Check sheet for the modelled part. Datum: model origin and axes. Units: mm. A direction names the side the tool comes from. Coordinates: 2 decimals unless noted, no trailing zeros. Loops run counter-clockwise (first coordinate to the right, second up) from the corner with the lowest first, then second, coordinate; pieces in that order, holes last. Notation, with made-up numbers: M -36.5,10 L -9.5,10 A21 ccw -9.5,14 Z; hole C 61.25,51 d5. An arc over 180 degrees is marked long. Use CSV: the item, a comma, the result in double quotes. Start each with the question number.
(1) Set-up check for faces 1 (the cylindrical face through (-61.922, -104.907, 3.944)), 2 (the flat face through (-2, 120, 4)): record each of +Z, -Z, +X, -X, +Y, -Y from which the full face is reachable in a straight line by a thin tool's end or side.
(2) Scan lines: line 1 (Y direction, x = 98.5, z = 7.75); line 2 (X direction, y = 79, z = 3); line 3 (X direction, y = 106, z = 5). Record each from-to range of solid material in increasing order.
(3) Section check B-B on y = -105. Record the cut outline in (x, z).
(4) Go/stop test with a flat-tipped pin: pin 1 Ø5.5 at (x, y) = (45.58, -77.36) entering from -Z. Record where the tip stops, or that it passes through.
(5) Section check D-D on x = -16. Record the cut outline in (y, z).
(6) Section check A-A on x = 97.5. Record the cut outline in (y, z), and give its area (3 significant figures).
(7) Section check C-C on y = 0. Record the cut outline in (x, z).
(8) Draft check along X on faces 3 (the cylindrical face through (-109.943, 104.907, 3.944)), 4 (the flat face through (-55, 55, 8)), 5 (the flat face through (119.579, -2, 4)). Enter one of: pulls with the +X half, pulls with the -X half, needs draft (parallel to the pull), parting line crosses it, or undercut.
from build123d import *

# Parameters (mm, degrees)
F0_W     = 240
F0_H     = 240
F0_R     = 4.5
F0_R_2   = 65
F1_DEPTH = 8


with BuildPart() as f1:
    # F0 (on Top) → F1 (new body)
    with BuildSketch(Plane.XY):
        with Locations((-0.42114, 0)):
            Rectangle(F0_W, F0_H)
        with BuildLine():
            ThreePointArc((-105.444208, -109.5), (-109.944211, -104.994235), (-105.432677, -100.500015))
            Line((-105.432677, -100.500015), (-66.432677, -100.500015))
            ThreePointArc((-66.432677, -100.500015), (-61.921144, -105.005765), (-66.444208, -109.499941))
            Line((-66.444208, -109.499941), (-105.444208, -109.5))
        make_face(mode=Mode.SUBTRACT)
        with Locations((-46.42114, -77.356318)):
            Circle(F0_R, mode=Mode.SUBTRACT)
        with Locations((45.57886, -77.356318)):
            Circle(F0_R, mode=Mode.SUBTRACT)
        with BuildLine():
            ThreePointArc((64.555792, -109.5), (60.055789, -104.994235), (64.567323, -100.500015))
            Line((64.567323, -100.500015), (103.567323, -100.500015))
            ThreePointArc((103.567323, -100.500015), (108.078856, -105.005765), (103.555792, -109.499941))
            Line((103.555792, -109.499941), (64.555792, -109.5))
        make_face(mode=Mode.SUBTRACT)
        with BuildLine():
            ThreePointArc((-105.444208, 100.5), (-109.944211, 105.005765), (-105.432677, 109.499985))
            Line((-105.432677, 109.499985), (-66.432677, 109.499985))
            ThreePointArc((-66.432677, 109.499985), (-61.921144, 104.994235), (-66.444208, 100.500059))
            Line((-66.444208, 100.500059), (-105.444208, 100.5))
        make_face(mode=Mode.SUBTRACT)
        with Locations((-46.42114, 77.356318)):
            Circle(F0_R, mode=Mode.SUBTRACT)
        with Locations((-0.42114, 0)):
            Circle(F0_R_2, mode=Mode.SUBTRACT)
        with Locations((45.57886, 77.356318)):
            Circle(F0_R, mode=Mode.SUBTRACT)
        with BuildLine():
            ThreePointArc((64.555792, 100.5), (60.055789, 105.005765), (64.567323, 109.499985))
            Line((64.567323, 109.499985), (103.567323, 109.499985))
            ThreePointArc((103.567323, 109.499985), (108.078856, 104.994235), (103.555792, 100.500059))
            Line((103.555792, 100.500059), (64.555792, 100.5))
        make_face(mode=Mode.SUBTRACT)
    extrude(amount=F1_DEPTH)


solid = f1.part
Outcome:
1,face 1,"+Z, -Z"
1,face 2,"+Z, -Z, +X, -X, +Y"
2,line 1,"y = -120 to -109.5, -100.5 to 100.5, 109.5 to 120"
2,line 2,"x = -120.42 to -50.61, -42.23 to 41.39, 49.77 to 119.58"
2,line 3,"x = -120.42 to -109.83, -62.03 to 60.17, 107.97 to 119.58"
3,outline,"M -120.42,0 L -109.94,0 L -109.94,8 L -120.42,8 Z; M -61.92,0 L 60.06,0 L 60.06,8 L -61.92,8 Z; M 108.08,0 L 119.58,0 L 119.58,8 L 108.08,8 Z"
4,pin 1,"passes through"
5,outline,"M -120,0 L -63.11,0 L -63.11,8 L -120,8 Z; M 63.11,0 L 120,0 L 120,8 L 63.11,8 Z"
6,outline,"M -120,0 L -109.5,0 L -109.5,8 L -120,8 Z; M -100.5,0 L 100.5,0 L 100.5,8 L -100.5,8 Z; M 109.5,0 L 120,0 L 120,8 L 109.5,8 Z"
6,area,"1,780 mm²"
7,outline,"M -120.42,0 L -65.42,0 L -65.42,8 L -120.42,8 Z; M 64.58,0 L 119.58,0 L 119.58,8 L 64.58,8 Z"
8,face 3,"undercut"
8,face 4,"needs draft"
8,face 5,"pulls with the +X half"
